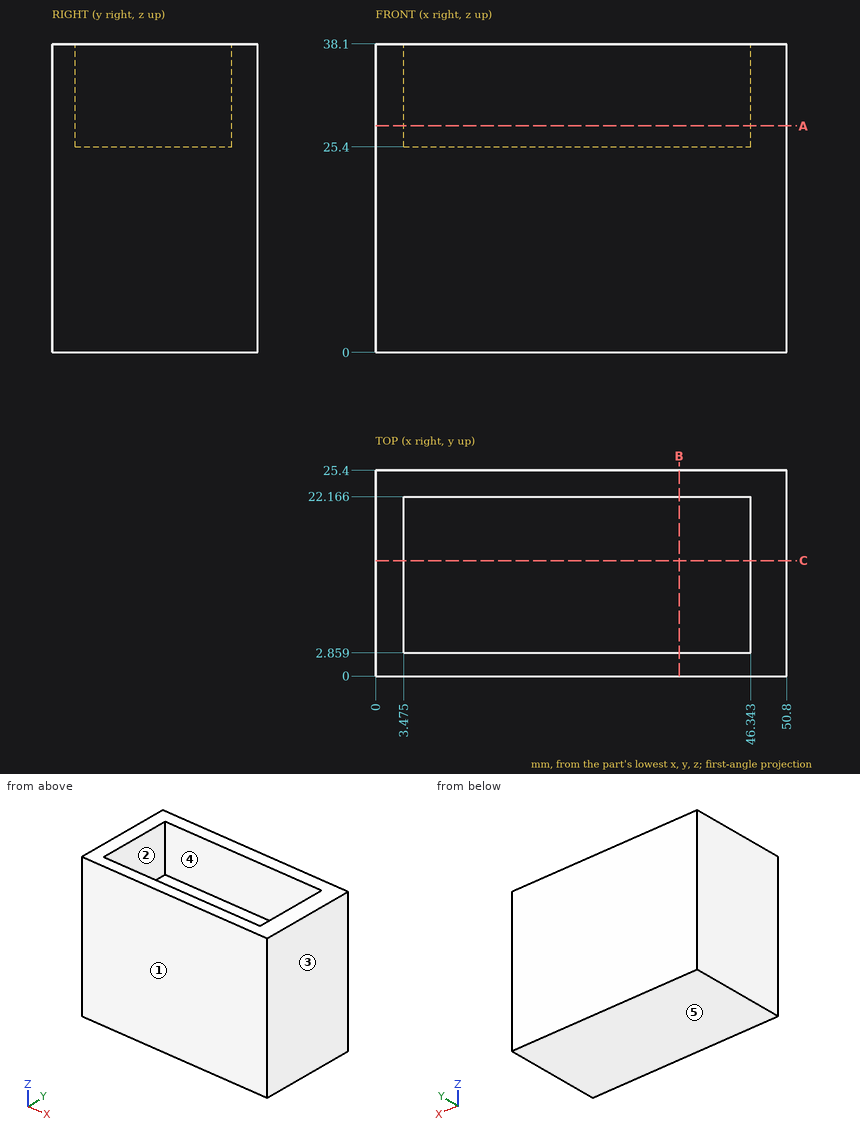
Study the drawing (mm; zero at the part's minimum x, y, z) and answer. A direction names the side the tool comes from. Round coordinates to 2 decimals unless told otherwise and drop trailing zeros. Write each loop counter-clockwise with the first axis right and the second up, starting at its lowest first coordinate (ties: lowest second). Pieces come first, ordered by that corner, then holes. Notation, with made-up numbers: (79.25, -3.75) - (136.25, -3.75) arc R11 cw to (136.25, 16.25) - close; hole circle Ø2 at (43, 15.25). An arc over 180 degrees is marked (long way). Return JSON: item names as keys, results as strings. Group by question number.
Q1. The part is cut by section C-C on y = 14.25. Write down the section's boundary in (x, z) (1 decimal).
Q2. Find the intervals of material crossed by L1, parallel to X at y = 5.5, z = 34.5 (1 decimal); L2, parallel to Y at x = 10, z = 36; L3, parallel to Z at x = 33.5, y = 17.75, in increasing order.
Q3. This flat-tipped pin is pushed along its axis until it touches: pin 1 Ø9.5 at (x, y) = (25.5, 10) entering from +Z. Where does it stop, or does it pass through?
Q4. The part is cut by section B-B on x = 37.5. Write down the section's boundary in (y, z).
Q5. The part is cut by section A-A on z = 28. Write down the section's boundary in (x, y) (1 decimal).
Q6. For the marked faces 1 and 2, determine the directions among +Z, -Z, +X, -X, +Y, -Y from which every point of the face is accessible in a straight line to the end or side of a thin tool.
Q7. The mould has two halves that part along X. Classify the marked faces 3, 4 and 5: released by +X, released by -X, zero draft, split by the parting line, or undercut.
Solved:
{
 "1": {"outline": "(0, 0) - (50.8, 0) - (50.8, 38.1) - (46.3, 38.1) - (46.3, 25.4) - (3.5, 25.4) - (3.5, 38.1) - (0, 38.1) - close"},
 "2": {"L1": "0 to 3.5, 46.3 to 50.8", "L2": "0 to 2.86, 22.17 to 25.4", "L3": "0 to 25.4"},
 "3": {"pin 1": "z = 25.4"},
 "4": {"outline": "(0, 0) - (25.4, 0) - (25.4, 38.1) - (22.17, 38.1) - (22.17, 25.4) - (2.86, 25.4) - (2.86, 38.1) - (0, 38.1) - close"},
 "5": {"outline": "(0, 0) - (50.8, 0) - (50.8, 25.4) - (0, 25.4) - close; hole (3.5, 2.9) - (46.3, 2.9) - (46.3, 22.2) - (3.5, 22.2) - close"},
 "6": {"face 1": "+Z, -Z, +X, -X, -Y", "face 2": "+Z"},
 "7": {"face 3": "released by +X", "face 4": "undercut", "face 5": "zero draft"}
}
